Autodesk Inventor part; units mm, degrees
ref_plane "YZ Plane" through (0, 0, 0) normal (1, 0, 0) x (0, 1, 0)
ref_plane "XZ Plane" through (0, 0, 0) normal (0, 1, 0) x (-1, 0, 0)
ref_plane "XY Plane" through (0, 0, 0) normal (0, 0, 1) x (1, 0, 0)
sketch "Эскиз1" plane through (0, 0, 0) normal (0, 1, 0) x (-1, 0, 0)
  line L0 (-21, 25) -> (21, 25)
  line L1 (25, 21) -> (25, -21)
  line L2 (21, -25) -> (-21, -25)
  line L3 (-25, -21) -> (-25, 21)
  line L4 (-25, 25) -> (25, -25) construction
  line L5 (25, 25) -> (-25, -25) construction
  line L6 (-11.5, -5) -> (11.5, -5)
  line L7 (11.5, -5) -> (11.5, 5)
  line L8 (11.5, 5) -> (-11.5, 5)
  line L9 (-11.5, 5) -> (-11.5, -5)
  line L10 (-11.5, -5) -> (11.5, 5) construction
  line L11 (11.5, -5) -> (-11.5, 5) construction
  line L12 (-3.5, 5) -> (-3.5, -5)
  line L13 (4, 5) -> (4, -5) construction
  circle A0 centre (4, 0) radius 7.25
  arc A1 (21, -25) -> (25, -21) centre (21, -21) ccw
  arc A2 (25, 21) -> (21, 25) centre (21, 21) ccw
  arc A3 (-21, 25) -> (-25, 21) centre (-21, 21) ccw
  arc A4 (-25, -21) -> (-21, -25) centre (-21, -21) ccw
  point P0 (0, 0)
  point P1 (-1.25, -5)
  point P2 (-1.25, 5)
  dimension "d0" = 50
  dimension "d1" = 50
  dimension "d2" = 23
  dimension "d3" = 10
  dimension "d4" = 8
  dimension "d29" = 7.5
  dimension "d30" = 14.5
  dimension "d52" = 4
extrude "Выдавливание13" add sketch "Эскиз1" along normal blind 15 contours L0 A2 L1 A1 L2 A4 L3 A3 | L6 A0 | A0 L8
sketch "Эскиз6" plane through (0, 0, 0) normal (0, -1, 0) x (1, 0, 0)
  line L0 (22.5, 22.5) -> (-22.5, 22.5)
  line L1 (-22.5, 22.5) -> (-22.5, -22.5)
  line L2 (-22.5, -22.5) -> (22.5, -22.5)
  line L3 (22.5, -22.5) -> (22.5, 22.5)
  line L4 (22.5, 22.5) -> (-22.5, -22.5) construction
  line L5 (-22.5, 22.5) -> (22.5, -22.5) construction
  point P0 (0, 0)
  dimension "d41" = 45
  dimension "d42" = 45
extrude "Выдавливание14" add sketch "Эскиз6" along normal blind 5
extrude "Выдавливание15" cut sketch "Эскиз1" against normal through all contours L12 L8 A0 L6 | A0 L8 L6 | A0 L8 L7 L6
sketch "Эскиз7" plane through (0, 15, 0) normal (0, 1, 0) x (1, 0, 0)
  circle A0 centre (-4.0005, 0) radius 7
  line L0 (21, 25) -> (-21, 25)
  line L1 (-25, 21) -> (-25, -21)
  point P0 (0, 0)
  point P1 (25, 25)
  point P2 (-25, 25)
  point P3 (-25, -25)
  dimension "d47" = 14
  dimension "d48" = 25
  dimension "d49" = 20.9995
extrude "Выдавливание16" cut sketch "Эскиз7" against normal blind 15
sketch "Эскиз8" plane through (0, -5, 0) normal (0, -1, 0) x (1, 0, 0)
  point P0 (0, 0)
sketch "Эскиз9" plane through (0, -5, 0) normal (0, -1, 0) x (1, 0, 0)
  point P0 (0, 0)
sketch "Эскиз10" plane through (0, -5, 0) normal (0, -1, 0) x (1, 0, 0)
  line L0 (-11.5, -7.3) -> (11, -7.3)
  line L1 (11, -7.3) -> (11, 7.3)
  line L2 (11, 7.3) -> (-11.5, 7.3)
  line L3 (-11.5, 7.3) -> (-11.5, -7.3)
  point P0 (0, 0)
  dimension "d53" = 11.5
  dimension "d54" = 14.6
  dimension "d55" = 7.3
  dimension "d56" = 22.5
extrude "Выдавливание17" cut sketch "Эскиз10" against normal blind 1
properties part number "platform"
Can you work these out from the model? Positions are in its coordinate system, mm. A direction names the side the tool comes from. Give positions to 0.01 mm unless a question says otherwise; leave off trailing zeros. Loops run counter-clockwise (first coordinate to the right, second up) from the corner with the lowest first, then second, coordinate; pieces in that order, holes last. Notation, with made-up numbers: (7, 10.25) - (46, 10.25) arc R9 ccw to (46, 22.25) - close; hole circle Ø11 at (8.5, 46). An arc over 180 degrees is marked (long way). Answer as a JSON object with one key per item and string values.
Q1. Which directions (+Z, -Z, +X, -X, +Y, -Y) give clear straight access to the entire face, cutting with the end or side of a thin tool? Please do faces 1 (the flat face through (-22.5, -2, 0)), 2 (the flat face through (3, 6, -5)), 3 (the flat face through (22.5, -2, 0)), 4 (the flat face through (3.5, -2, 0)).
Geometry says:
{"face 1": "+Z, -Z, -X, -Y", "face 2": "+Y", "face 3": "+Z, -Z, +X, -Y", "face 4": "+Y, -Y"}
Q2. Imagine slicing it at C-C on z = -9. Write out the boundary of the cut face in (x, y), plus the area to 3 significant figures.
Geometry says:
{"outline": "(-25, 0) - (-22.5, 0) - (-22.5, -5) - (22.5, -5) - (22.5, 0) - (25, 0) - (25, 15) - (-25, 15) - close", "area": "975 mm²"}
Q3. Imagine slicing it at D-D on y = 7.5. Write out the boundary of the cut face in (x, z), plus the area to 3 significant figures.
Geometry says:
{"outline": "(-25, -21) arc R4 ccw to (-21, -25) - (21, -25) arc R4 ccw to (25, -21) - (25, 21) arc R4 ccw to (21, 25) - (-21, 25) arc R4 ccw to (-25, 21) - close; hole (-11.5, -5) - (-8.9, -5) arc R7 ccw to (0.9, -5) - (11.5, -5) - (11.5, 5) - (0.9, 5) arc R7 ccw to (-8.9, 5) - (-11.5, 5) - close", "area": "2,230 mm²"}
Q4. If I drill on L1, parallel to Z at x = -8, y = -0.5; L2, parallel to X at y = -0.75, z = 3; L3, parallel to X at y = -4, z = 13, over which ranges is the centre line in solid material (lowest first)?
Geometry says:
{"L1": "-22.5 to -5, 5 to 22.5", "L2": "-22.5 to -11.5, 3.5 to 22.5", "L3": "-22.5 to 22.5"}
Q5. If we mould it in two halves opening along X, with no side actions, what happens to faces 5 (the flat face through (5, -4, 0)), 6 (the cylindrical face through (23.859, 7.395, 23.797)), 7 (the flat face through (0, 0, 24)), 8 (the flat face through (7, 0, 0))? For each: pulls with the +X half, pulls with the -X half, needs draft (parallel to the pull), parting line crosses it, or undercut.
Geometry says:
{"face 5": "undercut", "face 6": "pulls with the +X half", "face 7": "needs draft", "face 8": "undercut"}
Q6. Will these pins go through, and if not, where does the flat tip stop? P1, Ø5.5, axis at y = -3.5, z = 7, coming from the +X side; P2, Ø2, axis at y = -2.5, z = 1.5, coming from the -X side; P3, Ø1.1, axis at x = -4, y = -4.5, coming from the +Z side.
Geometry says:
{"P1": "x = 22.5", "P2": "x = -22.5", "P3": "z = 22.5"}
Q7. Imagine slicing it at A-A on y = -1.5. Write out the boundary of the cut face in (x, z), plus the area to 4 significant figures.
Geometry says:
{"outline": "(-22.5, -22.5) - (22.5, -22.5) - (22.5, 22.5) - (-22.5, 22.5) - close; hole (-11.5, -5) - (3.5, -5) - (3.5, 5) - (-11.5, 5) - close", "area": "1,875 mm²"}
Q8. Imagine slicing it at B-B on x = -6. Write out the boundary of the cut face in (y, z), plus the area to 3 significant figures.
Geometry says:
{"outline": "(-5, -22.5) - (0, -22.5) - (0, -25) - (15, -25) - (15, -6.71) - (0, -6.71) - (0, -5) - (-4, -5) - (-4, -7.3) - (-5, -7.3) - close; (-5, 7.3) - (-4, 7.3) - (-4, 5) - (0, 5) - (0, 6.71) - (15, 6.71) - (15, 25) - (0, 25) - (0, 22.5) - (-5, 22.5) - close", "area": "719 mm²"}
